The drawing under review shows one solid part. Ordinate dimensions are in mm from its lowest x, y, z. A direction names the side the tool comes from. Coordinates: 2 decimals unless noted, no trailing zeros. Write each loop counter-clockwise with the first axis right and the second up, starting at its lowest first coordinate (ties: lowest second). Pieces come first, ordered by that corner, then holes. Notation, with made-up numbers: M 57,62 L 111,62 A19 cw 111,66 Z; hole C 12,26.25 d11. An arc over 180 degrees is marked long. Answer as CSV lines item,"result". Start each with the question number.
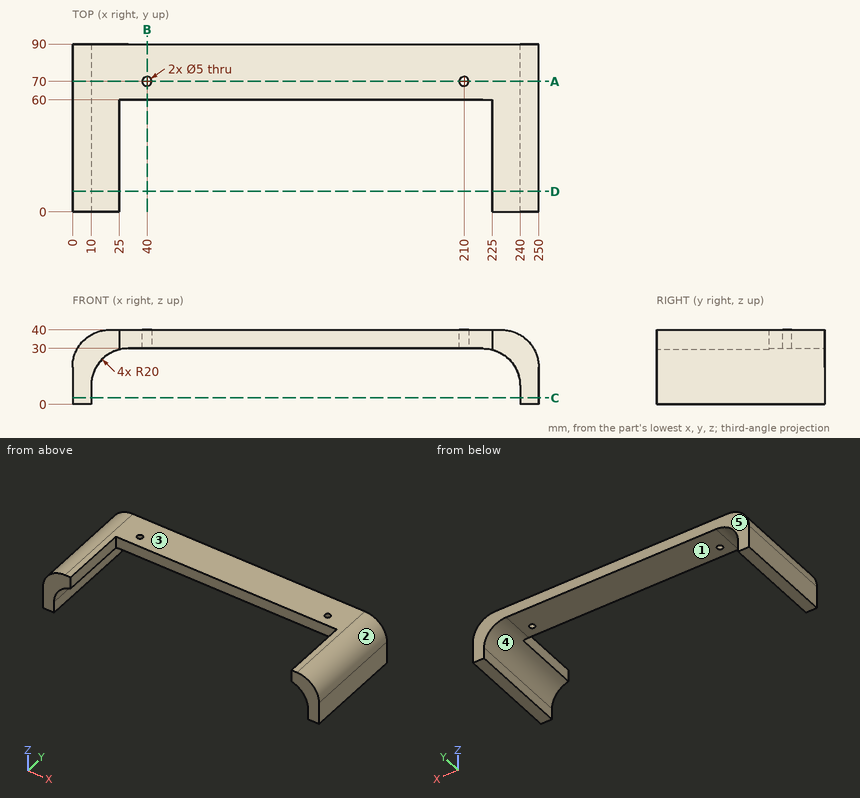
1) Tool access review of the marked faces 4 and 5: name each direction out of +Z, -Z, +X, -X, +Y, -Y from which nothing blocks a thin tool from reaching the whole face with its end or side.
2) To check wall thickness, follow line 1 (X direction, y = 54, z = 8.5); line 2 (Y direction, x = 40, z = 36); line 3 (X direction, y = 68, z = 31). State the ranges of each line that lie inside material, in increasing order. Write a range as [from, to].
3) Mouldability with a two-part tool opening along X and no side actions: class the marked faces 1, 2 and 3 as +X half, -X half, draft (parallel to the pull), parting line (faces both ways), or undercut.
4) Clearance check with flat-ended pins moving along their axes: pin 1 Ø9 at (x, y) = (96.5, 78.5) entering from -Z; pin 2 Ø8.5 at (y, z) = (19.5, 33) entering from +X; pin 3 Ø8.5 at (x, z) = (102.5, 35.5) entering from -Y. State where each tip first meets the part, or that it passes through.
5) Take a section at C-C on z = 3.5. Give the boundary of the cut face in (x, y).
6) Take a section at D-D on y = 11. Give the boundary of the cut face in (x, z).
7) Take a section at B-B on x = 40. Give the boundary of the cut face in (y, z), and give its area (3 significant figures).
8) Take a section at A-A on y = 70. Give the boundary of the cut face in (x, z).
Results:
1,face 4,"-Z, +Y, -Y"
1,face 5,"+Z, -Z, +X, -X, +Y"
2,line 1,"x = [0, 10], [240, 250]"
2,line 2,"y = [60, 67.5], [72.5, 90]"
2,line 3,"x = [3.3, 38.5], [41.5, 208.5], [211.5, 246.7]"
3,face 1,"undercut"
3,face 2,"+X half"
3,face 3,"draft"
4,pin 1,"stops at z = 30"
4,pin 2,"stops at x = 247.98"
4,pin 3,"stops at y = 60"
5,outline,"M 0,0 L 10,0 L 10,90 L 0,90 Z; M 240,0 L 250,0 L 250,90 L 240,90 Z"
6,outline,"M 0,0 L 10,0 L 10,10 A20 cw 25,29.36 L 25,40 L 20,40 A20 ccw 0,20 Z; M 225,29.36 A20 cw 240,10 L 240,0 L 250,0 L 250,20 A20 ccw 230,40 L 225,40 Z"
7,outline,"M 60,30 L 67.5,30 L 67.5,40 L 60,40 Z; M 72.5,30 L 90,30 L 90,40 L 72.5,40 Z"
7,area,"250 mm²"
8,outline,"M 0,0 L 10,0 L 10,10 A20 cw 30,30 L 37.5,30 L 37.5,40 L 20,40 A20 ccw 0,20 Z; M 42.5,30 L 207.5,30 L 207.5,40 L 42.5,40 Z; M 212.5,30 L 220,30 A20 cw 240,10 L 240,0 L 250,0 L 250,20 A20 ccw 230,40 L 212.5,40 Z"
